Part model, mm, in its own coordinate system. A direction names the side the tool comes from. Give positions to 0.01 mm unless a question says otherwise; leave off trailing zeros. Write each loop counter-clockwise with the first axis right and the second up, starting at its lowest first coordinate (ties: lowest second). Pieces come first, ordered by that corner, then holes. Notation, with made-up numbers: M 72,-24.5 L 121,-24.5 A23 cw 121,0.5 Z; hole C 58,-24 d6. An arc over 180 degrees is marked long. Write item = value, one per line. Start each with the question number.
Autodesk Inventor part; units mm, degrees
ref_plane "YZ Plane" through (0, 0, 0) normal (1, 0, 0) x (0, 1, 0)
ref_plane "XZ Plane" through (0, 0, 0) normal (0, 1, 0) x (-1, 0, 0)
ref_plane "XY Plane" through (0, 0, 0) normal (0, 0, 1) x (1, 0, 0)
sketch "Náčrt1" plane through (0, 0, 0) normal (0, 0, 1) x (1, 0, 0)
  line L0 (0, 0) -> (14, 0)
  line L1 (14, 0) -> (14, 25)
  line L2 (14, 25) -> (0, 25)
  line L3 (0, 25) -> (0, 0)
  circle A0 centre (7, 7) radius 2.5
  line L4 (0, 25) -> (14, 25)
  line L5 (14, 25) -> (14, 21)
  line L6 (14, 21) -> (0, 21)
  line L7 (0, 21) -> (0, 25)
  point P0 (0, 0)
  point P1 (7, 0)
  point P2 (0, 21)
  dimension "d0" = 14
  dimension "d1" = 25
  dimension "d2" = 5
  dimension "d3" = 7
  dimension "d4" = 7
  dimension "d5" = 4
extrude "Vysunutí1" add sketch "Náčrt1" against normal blind 4
extrude "Vysunutí2" add sketch "Náčrt1" along normal blind 60 contours L3 L2 L1 L6
sketch "Náčrt2" plane through (0, 25, -4) normal (0, 1, 0) x (1, 0, 0)
  point P0 (0, -4)
sketch "Náčrt3" plane through (0, 25, -4) normal (0, 1, 0) x (1, 0, 0)
  line L0 (14, 0) -> (14, -64)
  line L1 (0, 0) -> (14, 0)
  line L2 (0, 0) -> (0, -64)
  line L3 (14, -64) -> (0, -64)
  line L4 (7, -6.7883) -> (10.6, -8.8668)
  line L5 (9.075, -57.6142) -> (9.075, -11.0396)
  line L6 (10.6, -59.7938) -> (7, -61.8722)
  line L7 (7, -61.8722) -> (3.4, -59.7938)
  line L8 (7, -61.8722) -> (3.4, -59.7938)
  line L9 (10.6, -59.7938) -> (7, -61.8722)
  line L10 (7, -6.7883) -> (10.6, -8.8668)
  arc A0 (4.925, -57.693) -> (9.075, -57.6142) centre (7.0012, -57.7147) ccw
  arc A1 (4.925, -57.693) -> (9.075, -57.6142) centre (7.0012, -57.7147) ccw
  line L11 (4.925, -11.0876) -> (4.925, -57.693)
  line L12 (9.075, -57.6142) -> (9.075, -11.0396)
  line L13 (10.6, -8.8668) -> (10.6, -59.7938)
  line L14 (10.6, -8.8668) -> (10.6, -59.7938)
  line L15 (3.4, -59.7938) -> (3.4, -8.8668)
  line L16 (3.4, -59.7938) -> (3.4, -8.8668)
  arc A2 (9.075, -11.0396) -> (4.925, -11.0876) centre (6.9987, -10.9484) ccw
  arc A3 (9.075, -11.0396) -> (4.925, -11.0876) centre (6.9987, -10.9484) ccw
  line L17 (3.4, -8.8668) -> (7, -6.7883)
  line L18 (3.4, -8.8668) -> (7, -6.7883)
  line L19 (4.925, -11.0876) -> (4.925, -57.693)
  point P0 (0, -4)
  point P1 (7, -8.87)
  point P2 (7, -8.87)
  point P3 (7, -64)
  point P4 (7.0406, -59.7906)
  dimension "d10" = 4.15
  dimension "d11" = 2.1278
  dimension "d12" = 2.0816
  dimension "d13" = 1.525
extrude "Vysunutí3" cut sketch "Náčrt3" against normal blind 60 contours A0 L11 A2 L5
extrude "Vysunutí4" cut sketch "Náčrt3" against normal blind 2.5 contours L4 L13 L6 L7 L15 L17
fillet "Zaoblení1" radius 2 2 edges at (14, 23, 60) (0, 23, 60)
fillet "Zaoblení2" radius 2 2 edges at (14, 0, -2) (0, 0, -2)
fillet "Zaoblení3" radius 4 1 edges at (7, 21, 0)
properties part number "Sloupek" material "Olovo"
Q1. Two-plate mould, pull along Z, no slides. Class faces 4 (the face through (13.43, 0.6, -2.03)), 5 (the face through (13.4, 23.03, 59.43)), 6 (the face through (8.77, 23.77, 3.81)): +Z half, -Z half, draft (parallel to the pull), parting line (faces both ways), or undercut.
Q2. Tool access for faces 1 (the face through (4.925, 22, 30)), 2 (the face through (5.23, 23.77, 56.85)), 3 (the face through (7, 11, 0)): list every direction of +Z, -Z, +X, -X, +Y, -Y with a clear straight run to the whole face (end or side of a thin tool).
Q3. Drop flat-ended pins along their axis: P1, Ø5, axis at x = 6, z = 51.5, coming from the +Y side; P2, Ø4.5, axis at x = 7, y = 7, coming from the +Z side; P3, Ø1, axis at x = 3, z = 14.5, coming from the -Y side. Give the stop position or say it passes through.
Q4. Slice it at A-A (y = 7). Give the cut face in (x, z), and give its area (3 significant figures).
Q5. Slice it at D-D (x = 6.25). Give the cut face in (y, z).
Q6. Slice it at C-C (z = 18.5). Give the cut face in (x, y) (3 decimals), and give its area (3 significant figures).
Q7. Slice it at B-B (y = 21.75). Give the cut face in (x, z) (3 decimals).
Q8. Probe line 1 along Y through (x, z) = (7, -1.55); line 2 along X through (y, z) = (21.75, 43) (3 decimals); line 3 along Y through (x, z) = (10.5, 16). List the from-to ranges inside material, lowest first.
Working result:
q1.face_4 = draft
q1.face_5 = +Z half
q1.face_6 = undercut
q2.face_1 = +Y, -Y
q2.face_2 = +Y
q2.face_3 = +Z, +X, -X, -Y
q3.P1 = 22.5
q3.P2 = through
q3.P3 = 21
q4.outline = M 0,-4 L 4.5,-4 L 4.5,0 L 0,0 Z; M 9.5,-4 L 14,-4 L 14,0 L 9.5,0 Z
q4.area = 36.0 mm2
q5.outline = M 0,-4 L 4.62,-4 L 4.62,0 L 0,0 Z; M 9.38,-4 L 25,-4 L 25,3.22 L 22.5,3.22 L 22.5,5.01 L 21,5.01 L 21,4 A4 cw 17,0 L 9.38,0 Z; M 21,55.65 L 22.5,55.65 L 22.5,57.44 L 25,57.44 L 25,60 L 21,60 Z
q6.outline = M 0,21 L 4.925,21 L 4.925,22.5 L 3.4,22.5 L 3.4,25 L 0,25 Z; M 9.075,21 L 14,21 L 14,25 L 10.6,25 L 10.6,22.5 L 9.075,22.5 Z
q6.area = 31.8 mm2
q7.outline = M 0,-4 L 14,-4 L 14,58 A2 ccw 12,60 L 2,60 A2 ccw 0,58 Z; hole M 4.925,7.088 A2.078 ccw long 9.075,7.04 L 9.075,53.614 A2.076 ccw long 4.925,53.693 Z
q8.line_1 = 0 to 4.5, 9.5 to 25
q8.line_2 = 0 to 4.925, 9.075 to 14
q8.line_3 = 21 to 22.5
